The model under review builds one solid part; all positions refer to its coordinate system, in mm. Face numbers are marked on the shaded views. A direction names the side the tool comes from. Round coordinates to 2 decimals unless told otherwise and drop trailing zeros. Loops run counter-clockwise (first coordinate to the right, second up) from the corner with the lowest first, then second, coordinate; pieces in that order, holes last. Notation, with made-up numbers: (55.5, -39) -> (103.5, -39) arc R8 cw to (103.5, -35) -> close; hole circle Ø2 at (81.5, -4.75). An arc over 180 degrees is marked (long way). Use a Markdown table: item, result. Add a question column.
1) Wall thickness on probe 1 along X at (y, z) = (3.5, -6.75); probe 2 along Y at (x, z) = (-2, 12.5); probe 3 along X at (y, z) = (-197, 0.75): over which ranges is each line inside the solid? List them lowest first.
2) Consider section B-B on y = 97.5. Give the boundary of the cut face in (x, z), plus the area to 3 significant figures.
3) For the marked faces 1, 2 and 3, list the 3-axis set-ups (+Z, -Z, +X, -X, +Y, -Y) from which the entire face can be reached by the end or side of a thin tool; tool diameter is ignored.
4) Insertion check: pin 1 (3 mm diameter, centred on x = -3, y = 121.5, fed in from -Z); pin 2 (7.5 mm diameter, centred on y = -40, z = -2, fed in from -X); pin 3 (16.5 mm diameter, centred on y = -8, z = -3, fed in from +X). Each pin has a flat end and moves straight along its axis. Give the tip position at first contact, or say it passes through.
5) Consider section A-A on x = 0. Give the boundary of the cut face in (y, z), plus the area to 3 significant figures.
from build123d import *

# Parameters (mm, degrees)
F3_DEPTH = 35
F5_START = -5
F5_DEPTH = 355


with BuildPart() as f1:
    # F0 (on Right) → F1 (revolve)
    with BuildSketch(Plane.YZ):
        Polygon((-185, 0), (-185, 12.5), (-214, 12.5), (-214, 11.9), (-215.3, 11.9), (-215.3, 12.5), (-302, 12.5), (-302, 0), align=None)
        Polygon((185, 12.5), (185, 15), (-185, 15), (-185, 12.5), (-185, 0), (185, 0), align=None)
        Polygon((214, 12.5), (185, 12.5), (185, 0), (218, 0), (218, 12.5), (215.3, 12.5), (215.3, 11.9), (214, 11.9), align=None)
    revolve(axis=Axis((0, -30.9201925993, 0), (0, 1, 0)))

    # F2 (on face) → F3 (cut)
    with BuildSketch(Plane.XZ.offset(302)):
        with BuildLine():
            Line((-10.5, -6.7823299831), (-10.5, 6.7823299831))
            ThreePointArc((-10.5, 6.7823299831), (-12.5, 0), (-10.5, -6.7823299831))
        make_face()
        with BuildLine():
            ThreePointArc((12.5, 0), (11.9895788083, 3.5355339059), (10.5, 6.7823299831))
            Line((10.5, 6.7823299831), (10.5, -6.7823299831))
            ThreePointArc((10.5, -6.7823299831), (11.9895788083, -3.5355339059), (12.5, 0))
        make_face()
    extrude(amount=-F3_DEPTH, mode=Mode.SUBTRACT)

    # F4 (on face) → F5 (cut)
    with BuildSketch(Plane(origin=(0, 185, 0), x_dir=(-1, 0, 0), z_dir=(0, 1, 0)).offset(F5_START)):
        with BuildLine():
            Line((-13, -7.4833147735), (-13, 7.4833147735))
            ThreePointArc((-13, 7.4833147735), (-15, 0), (-13, -7.4833147735))
        make_face()
        with BuildLine():
            ThreePointArc((13, -7.4833147735), (15, 0), (13, 7.4833147735))
            Line((13, 7.4833147735), (13, -7.4833147735))
        make_face()
    extrude(amount=-F5_DEPTH, mode=Mode.SUBTRACT)


solid = f1.part
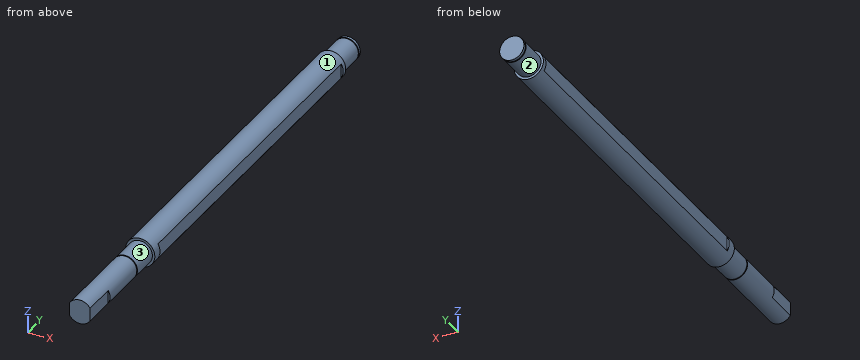
Result set:
| question | item | result |
|---|---|---|
| 1 | probe 1 | -13 to 13 |
| 1 | probe 2 | -185 to 185 |
| 1 | probe 3 | -12.48 to 12.48 |
| 2 | outline | (-13, -7.48) arc R15 ccw to (13, -7.48) -> (13, 7.48) arc R15 ccw to (-13, 7.48) -> close |
| 2 | area | 666 mm2 |
| 3 | face 1 | +Y, -Y |
| 3 | face 2 | +Y |
| 3 | face 3 | -Y |
| 4 | pin 1 | z = -14.92 |
| 4 | pin 2 | x = -13 |
| 4 | pin 3 | x = 13 |
| 5 | outline | (-302, -12.5) -> (-215.3, -12.5) -> (-215.3, -11.9) -> (-214, -11.9) -> (-214, -12.5) -> (-185, -12.5) -> (-185, -15) -> (185, -15) -> (185, -12.5) -> (214, -12.5) -> (214, -11.9) -> (215.3, -11.9) -> (215.3, -12.5) -> (218, -12.5) -> (218, 12.5) -> (215.3, 12.5) -> (215.3, 11.9) -> (214, 11.9) -> (214, 12.5) -> (185, 12.5) -> (185, 15) -> (-185, 15) -> (-185, 12.5) -> (-214, 12.5) -> (-214, 11.9) -> (-215.3, 11.9) -> (-215.3, 12.5) -> (-302, 12.5) -> close |
| 5 | area | 14,800 mm2 |
